Part model, mm, in its own coordinate system. Face numbers are marked on the shaded views. A direction names the side the tool comes from. Round coordinates to 2 decimals unless told otherwise and drop trailing zeros. Loops run counter-clockwise (first coordinate to the right, second up) from the corner with the lowest first, then second, coordinate; pieces in that order, holes last. Notation, with made-up numbers: (-17.5, -28) -> (2.5, -28) arc R22 cw to (2.5, -8) -> close; hole circle Ø11 at (-2, 75.25). An arc over 180 degrees is marked (long way). Use a Markdown table: item, result. Add a question column.
Item 1: Cut at B-B, the plane x = 32.5. List the corners of the cut face in (y, z), plus the area to 3 significant figures.
Item 2: Flat gauge pins, fed straight in: pin 1 (3 mm diameter, centred on x = 30.5, z = 6.5, fed in from +Y); pin 2 (5 mm diameter, centred on x = 62, z = 6, fed in from +Y); pin 3 (0.5 mm diameter, centred on y = -0.5, z = 6, fed in from -X). Where does each tip first touch, or does it go through?
Item 3: Probe line 1 (X direction, y = 2.5, z = 8.25); line 2 (Y direction, x = 10.5, z = 6.75); line 3 (X direction, y = 1.25, z = 3.25). List the from-to ranges inside material, lowest first. Write a range as [from, to].
Item 4: Cut at C-C, the plane x = 50.5. List the corners of the cut face in (y, z), plus the area to 3 significant figures.
Item 5: Cut at A-A, the plane z = 1.5. List the corners of the cut face in (x, y).
Item 6: Which spindle directions (+Z, -Z, +X, -X, +Y, -Y) get a long thin tool onto all of the face, cutting with end or side? Do the marked faces 1 and 2. Say none if no direction does.
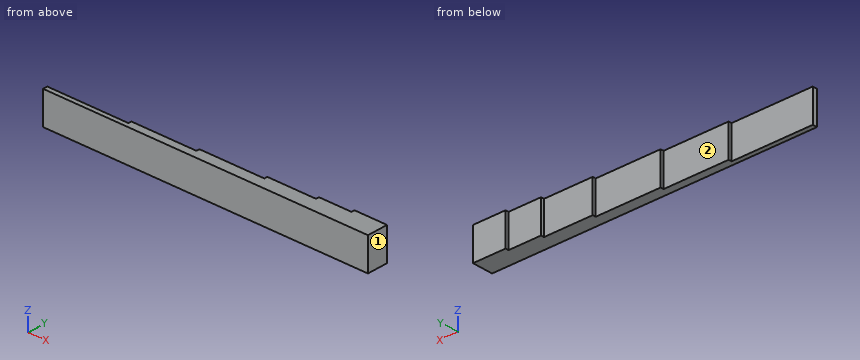
```python
from build123d import *

# Parameters (mm, degrees)
BOSS_EXTRUDE2_DEPTH = 10


with BuildPart() as part:
    # Sketch2 → Boss-Extrude2 (new body)
    with BuildSketch(Plane.XY):
        Polygon((20, 0), (0, 0), (0, -1), (-25, -1), (-25, -2.421519289), (75, -2.421519289), (75, 4), (65, 4), (65, 3), (55, 3), (55, 2), (40, 2), (40, 1), (20, 1), align=None)
    extrude(amount=BOSS_EXTRUDE2_DEPTH)


solid = part.part
```
A:
| question | item | result |
|---|---|---|
| 1 | outline | (-2.42, 0) -> (1, 0) -> (1, 10) -> (-2.42, 10) -> close |
| 1 | area | 34.2 mm^2 |
| 2 | pin 1 | stops at y = 1 |
| 2 | pin 2 | stops at y = 3 |
| 2 | pin 3 | stops at x = 0 |
| 3 | line 1 | x = [55, 75] |
| 3 | line 2 | y = [-2.42, 0] |
| 3 | line 3 | x = [40, 75] |
| 4 | outline | (-2.42, 0) -> (2, 0) -> (2, 10) -> (-2.42, 10) -> close |
| 4 | area | 44.2 mm^2 |
| 5 | outline | (-25, -2.42) -> (75, -2.42) -> (75, 4) -> (65, 4) -> (65, 3) -> (55, 3) -> (55, 2) -> (40, 2) -> (40, 1) -> (20, 1) -> (20, 0) -> (0, 0) -> (0, -1) -> (-25, -1) -> close |
| 6 | face 1 | +Z, -Z, +X, +Y, -Y |
| 6 | face 2 | +Z, -Z, -X, +Y |
